Input: part model. Units: mm. Frame: model coordinates. A direction names the side the tool comes from. Coordinates: 2 decimals unless noted, no trailing zeros. Order: outer loops, then holes, each group sorted by start corner. A loop starts at its lowest first (then second) coordinate and runs counter-clockwise, first axis right, second up. Notation, with made-up numbers: (70.5, 73) - (117.5, 73) arc R25 ccw to (117.5, 90) - close; hole circle Ø2 at (-32, -9.5). An arc over 180 degrees is marked (long way). One line per question, with ' | ' between items. Start each with the question number.
Autodesk Inventor part; units mm, degrees
ref_plane "YZ Plane" through (0, 0, 0) normal (1, 0, 0) x (0, 1, 0)
ref_plane "XZ Plane" through (0, 0, 0) normal (0, 1, 0) x (-1, 0, 0)
ref_plane "XY Plane" through (0, 0, 0) normal (0, 0, 1) x (1, 0, 0)
sketch "Эскиз4" plane through (0, 0, 0) normal (0, 0, 1) x (1, 0, 0)
  line L0 (0, 0) -> (20, 0)
  line L1 (20, 0) -> (20, 25)
  line L2 (16, 29) -> (4, 29)
  line L3 (0, 25) -> (0, 0)
  line L4 (4, 29) -> (0, 25)
  line L5 (16, 29) -> (20, 25)
  point P0 (20, 29)
  point P1 (0, 29)
  dimension "d20" = 20
  dimension "d21" = 29
  dimension "d22" = 4
  dimension "d23" = 4
  dimension "d24" = 4
  dimension "d25" = 4
revolve "Вращение3" add sketch "Эскиз4" angle 360 about axis through (0, 0, 0) along (1, 0, 0)
sketch "Эскиз5" plane through (0, 0, 0) normal (0, 0, 1) x (1, 0, 0)
  line L0 (0, 4) -> (9, 4)
  line L1 (9, 4) -> (9, -4)
  line L2 (9, -4) -> (0, -4)
  line L3 (0, -4) -> (0, 4)
  point P0 (0, 0)
  point P1 (0, 0)
  dimension "d27" = 9
  dimension "d28" = 8
extrude "Выдавливание2" cut sketch "Эскиз5" along normal through all both and the other way through all
sketch "Эскиз6" plane through (20, 0, 0) normal (1, 0, 0) x (0, 0, -1)
  point P0 (0, 0)
  point P1 (0, 0)
hole "Отверстие1" at (20, 0, 0) direction (-1, 0, 0) diameter 8 depth 6
sketch "Эскиз7" plane through (14, 0, 0) normal (1, 0, 0) x (0, 0, -1)
  circle A0 centre (0, 0) radius 4.5
  dimension "d38" = 9
extrude "Выдавливание3" cut sketch "Эскиз7" against normal blind 0.5
thread "Резьба3"
properties part number "711133"
(1) Section C-C (y = 0). Output: boundary loops of the cut face in (x, z).
(2) Draft query along Y for faces 4 (the face through (19.75, -5.47, 24.65)), 5 (the face through (9, 0, 0)), 6 (the face through (0, 12, 0)), 7 (the face through (16.958, 3.905, 0.867)). Return one class per face: +Y half, -Y half, draft (parallel to the pull), parting line (faces both ways), or undercut.
(3) Section B-B (x = 7.75). Output: boundary loops of the cut face in (y, z).
(4) Section D-D (x = 12). Output: boundary loops of the cut face in (y, z), then the cut area to 3 significant figures.
(5) Section A-A (z = 0). Output: boundary loops of the cut face in (x, y), then the cut area to 3 significant figures.
(6) Material intervals for line 1 along Y through (x, z) = (13.6, 0); line 2 along Y through (x, z) = (15.9, 0); line 3 along Z through (x, y) = (18.3, 0), sorted ascending. Write a range as from..to.
(7) Reachability of faces 1 (the face through (13.5, 0, 0)), 2 (the face through (0.25, -25.245, 0.506)), 3 (the face through (4, 4, 0)) from +Z, -Z, +X, -X, +Y, -Y: full face, straight path, thin tool, end or side. Return the list, or none.
(8) Pin query (flat end, axial travel): pin 1 (8 mm diameter, centred on x = 4, y = -7, fed in from +Z); pin 2 (2.5 mm diameter, centred on x = 5.5, z = 3, fed in from +Y); pin 3 (4.5 mm diameter, centred on y = 2, z = 0.5, fed in from +X); pin 4 (6.5 mm diameter, centred on y = 0, z = 0, fed in from +X). Return the tip coordinate at first contact, or that it passes through.
Worked answers:
1) outline: (9, -29) - (16, -29) - (20, -25) - (20, -4) - (14, -4) - (14, -4.5) - (13.5, -4.5) - (13.5, 4.5) - (14, 4.5) - (14, 4) - (20, 4) - (20, 25) - (16, 29) - (9, 29) - close
2) face 4: parting line | face 5: undercut | face 6: draft | face 7: undercut
3) outline: (-4, -28.72) - (-4, 28.72) arc R29 ccw to start; (4, -28.72) arc R29 ccw to (4, 28.72) - close
4) outline: circle Ø58 at (0, 0) | area: 2,640 mm²
5) outline: (0, -25) - (4, -29) - (16, -29) - (20, -25) - (20, -4) - (14, -4) - (14, -4.5) - (13.5, -4.5) - (13.5, 4.5) - (14, 4.5) - (14, 4) - (20, 4) - (20, 25) - (16, 29) - (4, 29) - (0, 25) - (0, 4) - (9, 4) - (9, -4) - (0, -4) - close | area: 1,000 mm²
6) line 1: y = -29..-4.5, 4.5..29 | line 2: y = -29..-4, 4..29 | line 3: z = -26.7..-4, 4..26.7
7) face 1: none | face 2: -X, -Y | face 3: +Z, -Z, -X
8) pin 1: stops at z = 28.72 | pin 2: stops at y = 28.95 | pin 3: stops at x = 20 | pin 4: stops at x = 13.5
